For this review, take the finished solid that the model builds, in its own axes (mm). Coordinates: 2 decimals unless noted, no trailing zeros. Order: outer loops, then holes, each group sorted by start corner. A loop starts at its lowest first (then second) coordinate and runs counter-clockwise, first axis right, second up. Notation, with made-up numbers: M 27,12.25 L 63,12.25 A24 ccw 63,46.25 Z; hole C 26,9.25 d6. An arc over 180 degrees is marked long. Use CSV: the item, a comma, the result in double quotes.
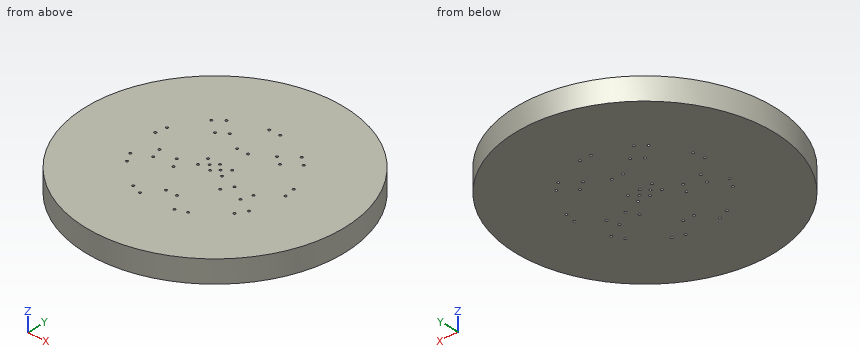
```python
from build123d import *

# Parameters (mm, degrees)
SCHIZZO1_R                   = 28.8
ESTRUSIONE_ESTRUSIONE1_DEPTH = 5
SCHIZZO2_R                   = 0.2635
TAGLIO_ESTRUSIONE1_DEPTH     = 6
RIPETIZIONECIRCOLARE1_COUNT  = 9
SCHIZZO6_R                   = 0.2635
TAGLIO_ESTRUSIONE2_DEPTH     = 6
RIPETIZIONECIRCOLARE2_COUNT  = 5
SCHIZZO7_R                   = 0.2635
TAGLIO_ESTRUSIONE3_DEPTH     = 6
RIPETIZIONECIRCOLARE3_COUNT  = 3
SCHIZZO8_R                   = 0.2635
TAGLIO_ESTRUSIONE4_DEPTH     = 6
RIPETIZIONECIRCOLARE4_COUNT  = 2
SCHIZZO9_R                   = 0.2545
TAGLIO_ESTRUSIONE5_DEPTH     = 6


with BuildPart() as part:
    # Schizzo1 → Estrusione-Estrusione1 (new body)
    with BuildSketch(Plane.XY):
        Circle(SCHIZZO1_R)
    extrude(amount=ESTRUSIONE_ESTRUSIONE1_DEPTH)

    # Schizzo2 → Taglio-Estrusione1 (cut, through all)
    with BuildSketch(Plane.XY.offset(5)):
        with Locations((-1.25, 14.79729705)):
            Circle(SCHIZZO2_R)
        with Locations((1.25, 14.79729705)):
            Circle(SCHIZZO2_R)
    taglio_estrusione1 = extrude(amount=-TAGLIO_ESTRUSIONE1_DEPTH, mode=Mode.SUBTRACT)

    # RipetizioneCircolare1: Taglio-Estrusione1 ×9 about axis
    ripetizionecircolare1_axis = Axis((0, -0.002477772, 0), (0, 0, 1))
    for i in range(1, RIPETIZIONECIRCOLARE1_COUNT):
        add(taglio_estrusione1.rotate(ripetizionecircolare1_axis, i * 360 / RIPETIZIONECIRCOLARE1_COUNT), mode=Mode.SUBTRACT)

    # Schizzo6 → Taglio-Estrusione2 (cut, through all)
    with BuildSketch(Plane.XY.offset(5)):
        with Locations((-1.25, -10.828088474)):
            Circle(SCHIZZO6_R)
        with Locations((1.25, -10.828088474)):
            Circle(SCHIZZO6_R)
    taglio_estrusione2 = extrude(amount=-TAGLIO_ESTRUSIONE2_DEPTH, mode=Mode.SUBTRACT)

    # RipetizioneCircolare2: Taglio-Estrusione2 ×5 about axis
    ripetizionecircolare2_axis = Axis((0, 0.001819614, 0), (0, 0, 1))
    for i in range(1, RIPETIZIONECIRCOLARE2_COUNT):
        add(taglio_estrusione2.rotate(ripetizionecircolare2_axis, i * 360 / RIPETIZIONECIRCOLARE2_COUNT), mode=Mode.SUBTRACT)

    # Schizzo7 → Taglio-Estrusione3 (cut, through all)
    with BuildSketch(Plane.XY.offset(5)):
        with Locations((-1.25, 6.836665854)):
            Circle(SCHIZZO7_R)
        with Locations((1.25, 6.836665854)):
            Circle(SCHIZZO7_R)
    taglio_estrusione3 = extrude(amount=-TAGLIO_ESTRUSIONE3_DEPTH, mode=Mode.SUBTRACT)

    # RipetizioneCircolare3: Taglio-Estrusione3 ×3 about axis
    ripetizionecircolare3_axis = Axis((0, -0.001145258, 0), (0, 0, 1))
    for i in range(1, RIPETIZIONECIRCOLARE3_COUNT):
        add(taglio_estrusione3.rotate(ripetizionecircolare3_axis, i * 360 / RIPETIZIONECIRCOLARE3_COUNT), mode=Mode.SUBTRACT)

    # Schizzo8 → Taglio-Estrusione4 (cut, through all)
    with BuildSketch(Plane.XY.offset(5)):
        with Locations((2.727178029, 1.25)):
            Circle(SCHIZZO8_R)
        with Locations((2.727178029, -1.25)):
            Circle(SCHIZZO8_R)
    taglio_estrusione4 = extrude(amount=-TAGLIO_ESTRUSIONE4_DEPTH, mode=Mode.SUBTRACT)

    # RipetizioneCircolare4: Taglio-Estrusione4 ×2 about axis
    ripetizionecircolare4_axis = Axis((-0.000457963, 2.794e-06, 0), (0, 0, 1))
    for i in range(1, RIPETIZIONECIRCOLARE4_COUNT):
        add(taglio_estrusione4.rotate(ripetizionecircolare4_axis, i * 360 / RIPETIZIONECIRCOLARE4_COUNT), mode=Mode.SUBTRACT)

    # Schizzo9 → Taglio-Estrusione5 (cut, through all)
    with BuildSketch(Plane.XY.offset(5)):
        with Locations((-1.25, 0)):
            Circle(SCHIZZO9_R)
        with Locations((1.25, 0)):
            Circle(SCHIZZO9_R)
        with Locations((0, -1.25)):
            Circle(SCHIZZO9_R)
        with Locations((0, 1.25)):
            Circle(SCHIZZO9_R)
    extrude(amount=-TAGLIO_ESTRUSIONE5_DEPTH, mode=Mode.SUBTRACT)


solid = part.part
```
Item 1: Add section A-A on x = -23. State the section outline as (y, z) points, and give its area (3 significant figures).
Solutions:
outline,"M -17.33,0 L 17.33,0 L 17.33,5 L -17.33,5 Z"
area,"173 mm^2"
Item 2: Add section C-C on y = 20. State the section outline as (x, z) points.
Solutions:
outline,"M -20.72,0 L 20.72,0 L 20.72,5 L -20.72,5 Z"
Item 3: To check wall thickness, follow line 1 along Y through (x, z) = (1.25, 1.9); line 2 along Y through (x, z) = (-15, 0.8); line 3 along Y through (x, z) = (17, 2.4). State the ranges of each line that lie inside material, in increasing order. Write a range as [from, to].
Solutions:
line 1,"[-28.77, -11.09], [-10.56, -0.25], [0.25, 6.57], [7.1, 14.53], [15.06, 28.77]"
line 2,"[-24.59, 1.17], [1.5, 24.59]"
line 3,"[-23.25, 23.25]"
Item 4: Clearance check with flat-ended pins moving along their axes: pin 1 Ø2 at (y, z) = (5.5, 2) entering from -X; pin 2 Ø1 at (y, z) = (-6, 4.5) entering from +X; pin 3 Ø3 at (x, z) = (-18.5, 4.5) entering from -Y. State where each tip first meets the part, or that it passes through.
Solutions:
pin 1,"x = -28.45"
pin 2,"x = 28.27"
pin 3,"y = -23.25"
Item 5: Add section B-B on z = 1.2. State how many separate pieces and enclosed holes the cut face has, and give its area (3 significant figures).
Solutions:
separate pieces,"1"
enclosed holes,"42"
area,"2,600 mm^2"
